Geometry: final body of the model. Coordinates: model frame, mm. Face numbers are marked on the shaded views. A direction names the side the tool comes from. Give positions to 0.01 mm unless a question says otherwise; leave off trailing zeros. Write each loop counter-clockwise with the first axis right and the second up, starting at its lowest first coordinate (ties: lowest second). Pieces come first, ordered by that corner, then holes. Notation, with made-up numbers: M 58,81 L 99,81 A22 ccw 99,114 Z; hole C 12.25,83 d1. An arc over 180 degrees is marked long. Answer as a JSON object with one key per item and string values.
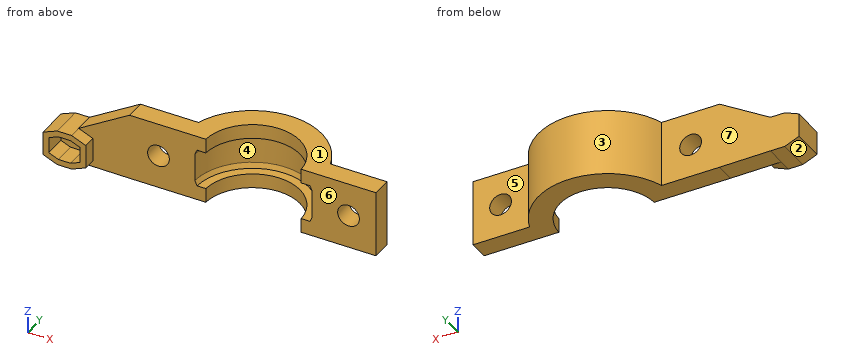
from build123d import *

# Parameters (mm, degrees)
REVOLVE_1_ANGLE       = 180
SKETCH_3_W            = 9
SKETCH_3_H            = 9.2
SKETCH_3_R            = 1.5
EXTRUDE_2_DEPTH       = 3
MOVE_FACE_1_OUTLINE_W = 34.2
MOVE_FACE_1_OUTLINE_H = 9.2
MOVE_FACE_1_OUTLINE_R = 1.5
MOVE_FACE_1_DEPTH     = 0.3
EXTRUDE_3_DEPTH       = 2.7
EXTRUDE_4_DEPTH       = 4.45
EXTRUDE_5_DEPTH       = 1.45
MOVE_FACE_2_BY        = 0.2


# Read off the part's stored shape, not the designer's step: Переместить грань1
with BuildPart() as part:
    # Эскиз2 → Повернуть1 (revolve)
    with BuildSketch(Plane(origin=(0, 0, 0), x_dir=(1, 0, 0), z_dir=(0, 1, 0))):
        Polygon((6.583922431, -16.610594473), (6.583922431, -14.610594473), (9.583922431, -14.610594473), (9.583922431, -23.810594473), (6.583922431, -23.810594473), (6.583922431, -21.810594473), (7.783922431, -21.810594473), (8.1, -21.132763939), (8.1, -17.288425007), (7.783922431, -16.610594473), align=None)
    revolve(axis=Axis((0, 0, 1.686216313), (0, 0, 1)), revolution_arc=REVOLVE_1_ANGLE)

    # Эскиз3 → Бобышка-Вытянуть2 (add)
    # profile 1 of 2: a face of its own
    with BuildSketch(Plane(origin=(0, 0, 0), x_dir=(1, 0, 0), z_dir=(0, 1, 0))):
        with Locations((12.6, -19.210594473)):
            Rectangle(SKETCH_3_W, SKETCH_3_H)
        with Locations(Location((13.1, -19.210594473, 0), (0, 0, 270))):
            Circle(SKETCH_3_R, mode=Mode.SUBTRACT)
    # profile 2 of 2: a face of its own
    with BuildSketch(Plane(origin=(0, 0, 0), x_dir=(1, 0, 0), z_dir=(0, 1, 0))):
        with Locations((-12.6, -19.210594473)):
            Rectangle(SKETCH_3_W, SKETCH_3_H)
        with Locations(Location((-13.1, -19.210594473, 0), (0, 0, 90))):
            Circle(SKETCH_3_R, mode=Mode.SUBTRACT)
    extrude(amount=EXTRUDE_2_DEPTH)

    # Move Face 1 outline → Move Face 1 (cut)
    with BuildSketch(Plane(origin=(0, 0, 0), x_dir=(1, 0, 0), z_dir=(0, 1, 0))):
        with Locations((0, -19.210594473)):
            Rectangle(MOVE_FACE_1_OUTLINE_W, MOVE_FACE_1_OUTLINE_H)
        with Locations((-13.1, -19.210594473)):
            Circle(MOVE_FACE_1_OUTLINE_R, mode=Mode.SUBTRACT)
        with Locations((13.1, -19.210594473)):
            Circle(MOVE_FACE_1_OUTLINE_R, mode=Mode.SUBTRACT)
    extrude(amount=MOVE_FACE_1_DEPTH, mode=Mode.SUBTRACT)

    # Эскиз4 → Бобышка-Вытянуть3 (add)
    with BuildSketch(Plane(origin=(0, 3, 0), x_dir=(1, 0, 0), z_dir=(0, 1, 0))):
        Polygon((-24.11, -14.660594473), (-17.1, -14.610594473), (-17.1, -23.810594473), (-24.11, -19.560594473), (-26.09, -19.560594473), (-28.05, -18.743927806), (-28.05, -15.47726114), (-26.09, -14.660594473), align=None)
        Polygon((-27.25, -16.010594473), (-27.25, -18.210594473), (-25.93, -18.760594473), (-24.27, -18.760594473), (-22.95, -18.210594473), (-22.95, -16.010594473), (-24.27, -15.460594473), (-25.93, -15.460594473), align=None, mode=Mode.SUBTRACT)
    extrude(amount=-EXTRUDE_3_DEPTH)

    # Эскиз5 → Бобышка-Вытянуть4 (add)
    with BuildSketch(Plane(origin=(0, 3, 0), x_dir=(1, 0, 0), z_dir=(0, 1, 0))):
        Polygon((-28.05, -15.47726114), (-28.05, -18.743927806), (-26.09, -19.560594473), (-24.11, -19.560594473), (-22.15, -18.743927806), (-22.15, -15.47726114), (-24.11, -14.660594473), (-26.09, -14.660594473), align=None)
        Polygon((-27.25, -16.010594473), (-27.25, -18.210594473), (-25.93, -18.760594473), (-24.27, -18.760594473), (-22.95, -18.210594473), (-22.95, -16.010594473), (-24.27, -15.460594473), (-25.93, -15.460594473), align=None, mode=Mode.SUBTRACT)
    extrude(amount=-EXTRUDE_4_DEPTH)

    # Эскиз5<2> → Бобышка-Вытянуть5 (add)
    with BuildSketch(Plane(origin=(0, 3, 0), x_dir=(1, 0, 0), z_dir=(0, 1, 0))):
        Polygon((-25.93, -15.460594473), (-27.25, -16.010594473), (-27.25, -18.210594473), (-25.93, -18.760594473), (-24.27, -18.760594473), (-22.95, -18.210594473), (-22.95, -16.010594473), (-24.27, -15.460594473), align=None)
    extrude(amount=-EXTRUDE_5_DEPTH)

    # Move Face 2: a face moved inward by 0.2
    extrude(part.faces().sort_by_distance((17.1, 1.65, 19.210594473))[0], amount=MOVE_FACE_2_BY, dir=(-1, 0, 0), mode=Mode.SUBTRACT)


solid = part.part
1) Line query: line 1 (X direction, y = 0, z = 16.5); line 2 (X direction, y = 2.5, z = 18.5); line 3 (Y direction, x = -21.5, z = 20.75). Output: solid intervals per line, ascending. Write a range as from..to.
Geometry check:
{"line 1": "x = -28.05..-27.25, -22.95..-22.15", "line 2": "x = -28.05..-14.42, -11.78..-7.7, 7.7..11.78, 14.42..16.9", "line 3": "y = 0.3..3"}
2) Set-up query: the marked faces 5, 6 and 7. Return all of +Z, -Z, +X, -X, +Y, -Y with unobstructed straight access to the full face (end or side cutting, diameter ignored); none if empty.
Geometry check:
{"face 5": "+Z, -Z, +X, +Y", "face 6": "+Z, -Z, +X, -Y", "face 7": "+Z, -Z, -X, +Y"}
3) Cut plane A-A on x = -13.1. Return loops of the section in (y, z).
Geometry check:
{"outline": "M 0.3,14.61 L 3,14.61 L 3,17.71 L 0.3,17.71 Z; M 0.3,20.71 L 3,20.71 L 3,23.81 L 0.3,23.81 Z"}
4) Contact query for flat-ended pins moving along their axis: P1, Ø0.9, axis at y = -1, z = 16.5, coming from the +X side; P2, Ø1, axis at x = 4, z = 20.5, coming from the +Y side; P3, Ø5, axis at x = -13.1, z = 19.21, coming from the -Y side. Output: stop coordinate, or through.
Geometry check:
{"P1": "stops at x = -22.15", "P2": "stops at y = 8.92", "P3": "stops at y = 0.3"}
5) Cut plane B-B on x = -25. Return loops of the section in (y, z), and give its area (3 significant figures).
Geometry check:
{"outline": "M -1.45,14.66 L 3,14.66 L 3,19.56 L -1.45,19.56 L -1.45,18.76 L 1.55,18.76 L 1.55,15.46 L -1.45,15.46 Z", "area": "11.9 mm2"}
6) Pull-direction query (Z, two-part tool) for the marked faces 1, 2, 3 and 4; classes: pulls with the +Z half, pulls with the -Z half, needs draft (parallel to the pull), parting line crosses it, or undercut.
Geometry check:
{"face 1": "pulls with the +Z half", "face 2": "pulls with the -Z half", "face 3": "needs draft", "face 4": "undercut"}
7) Cut plane D-D on x = -20.5. Return loops of the section in (y, z), and give its area (3 significant figures).
Geometry check:
{"outline": "M 0.3,14.63 L 3,14.63 L 3,21.75 L 0.3,21.75 Z", "area": "19.2 mm2"}
